Check sheet for the modelled part. Datum: model origin and axes. Units: mm. Face numbers are marked on the shaded views. A direction names the side the tool comes from. Give positions to 0.01 mm unless a question says otherwise; leave off trailing zeros. Order: outer loops, then holes, each group sorted by start corner. A loop starts at its lowest first (then second) coordinate and runs counter-clockwise, first axis right, second up.
```python
from build123d import *

# Parameters (mm, degrees)
SKETCH1_R           = 1.35
BOSS_EXTRUDE1_DEPTH = 3
SKETCH1_3_W         = 89.4
SKETCH1_3_H         = 3
BOSS_EXTRUDE2_DEPTH = 24
CUT_EXTRUDE1_REACH  = 5
SKETCH3_R           = 1.5
SKETCH3_R_2         = 1.75
CUT_EXTRUDE2_START  = -3
SKETCH3_5_R         = 2.25
SKETCH3_5_R_2       = 1.5
CUT_EXTRUDE2_DEPTH  = 1


with BuildPart() as part:
    # Sketch1 → Boss-Extrude1 (new body)
    with BuildSketch(Plane.XY):
        Polygon((-32.2510699, 8.892599614), (-38.2510699, 2.892599614), (-38.2510699, 0.892599614), (51.1489301, 0.892599614), (51.1489301, 2.892599614), (45.1489301, 8.892599614), align=None)
        with Locations((-18.2510699, 4.092599614)):
            Circle(SKETCH1_R, mode=Mode.SUBTRACT)
        with Locations((31.1489301, 4.092599614)):
            Circle(SKETCH1_R, mode=Mode.SUBTRACT)
    extrude(amount=BOSS_EXTRUDE1_DEPTH)

    # Sketch1<3> → Boss-Extrude2 (add)
    with BuildSketch(Plane.XY):
        with Locations((6.4489301, -0.607400386)):
            Rectangle(SKETCH1_3_W, SKETCH1_3_H)
    extrude(amount=BOSS_EXTRUDE2_DEPTH)

    # Sketch3 → Cut-Extrude1 (cut, up to next)
    with BuildSketch(Plane(origin=(0, 0.892599614, 0), x_dir=(1, 0, 0), z_dir=(0, 1, 0)), mode=Mode.PRIVATE) as cut_extrude1_sk1:
        with Locations((48.6489301, -15)):
            Circle(SKETCH3_R)
    cut_extrude1_tool1 = extrude(cut_extrude1_sk1.sketch, amount=-CUT_EXTRUDE1_REACH, mode=Mode.PRIVATE) & part.part
    add(cut_extrude1_tool1.solids().sort_by_distance((48.64893, 0.8926, 15))[0], mode=Mode.SUBTRACT)
    # Sketch3 → Cut-Extrude1 (cut, up to next)
    with BuildSketch(Plane(origin=(0, 0.892599614, 0), x_dir=(1, 0, 0), z_dir=(0, 1, 0)), mode=Mode.PRIVATE) as cut_extrude1_sk2:
        with Locations((48.6489301, -21)):
            Circle(SKETCH3_R)
    cut_extrude1_tool2 = extrude(cut_extrude1_sk2.sketch, amount=-CUT_EXTRUDE1_REACH, mode=Mode.PRIVATE) & part.part
    add(cut_extrude1_tool2.solids().sort_by_distance((48.64893, 0.8926, 21))[0], mode=Mode.SUBTRACT)
    # Sketch3 → Cut-Extrude1 (cut, up to next)
    with BuildSketch(Plane(origin=(0, 0.892599614, 0), x_dir=(1, 0, 0), z_dir=(0, 1, 0)), mode=Mode.PRIVATE) as cut_extrude1_sk3:
        with Locations((-35.7510699, -15)):
            Circle(SKETCH3_R)
    cut_extrude1_tool3 = extrude(cut_extrude1_sk3.sketch, amount=-CUT_EXTRUDE1_REACH, mode=Mode.PRIVATE) & part.part
    add(cut_extrude1_tool3.solids().sort_by_distance((-35.75107, 0.8926, 15))[0], mode=Mode.SUBTRACT)
    # Sketch3 → Cut-Extrude1 (cut, up to next)
    with BuildSketch(Plane(origin=(0, 0.892599614, 0), x_dir=(1, 0, 0), z_dir=(0, 1, 0)), mode=Mode.PRIVATE) as cut_extrude1_sk4:
        with Locations((-35.7510699, -21)):
            Circle(SKETCH3_R)
    cut_extrude1_tool4 = extrude(cut_extrude1_sk4.sketch, amount=-CUT_EXTRUDE1_REACH, mode=Mode.PRIVATE) & part.part
    add(cut_extrude1_tool4.solids().sort_by_distance((-35.75107, 0.8926, 21))[0], mode=Mode.SUBTRACT)
    # Sketch3 → Cut-Extrude1 (cut, up to next)
    with BuildSketch(Plane(origin=(0, 0.892599614, 0), x_dir=(1, 0, 0), z_dir=(0, 1, 0)), mode=Mode.PRIVATE) as cut_extrude1_sk5:
        with Locations((44.5489301, -6.2)):
            Circle(SKETCH3_R_2)
    cut_extrude1_tool5 = extrude(cut_extrude1_sk5.sketch, amount=-CUT_EXTRUDE1_REACH, mode=Mode.PRIVATE) & part.part
    add(cut_extrude1_tool5.solids().sort_by_distance((44.54893, 0.8926, 6.2))[0], mode=Mode.SUBTRACT)
    # Sketch3 → Cut-Extrude1 (cut, up to next)
    with BuildSketch(Plane(origin=(0, 0.892599614, 0), x_dir=(1, 0, 0), z_dir=(0, 1, 0)), mode=Mode.PRIVATE) as cut_extrude1_sk6:
        with Locations((-31.6510699, -6.2)):
            Circle(SKETCH3_R_2)
    cut_extrude1_tool6 = extrude(cut_extrude1_sk6.sketch, amount=-CUT_EXTRUDE1_REACH, mode=Mode.PRIVATE) & part.part
    add(cut_extrude1_tool6.solids().sort_by_distance((-31.65107, 0.8926, 6.2))[0], mode=Mode.SUBTRACT)

    # Sketch3<5> → Cut-Extrude2 (cut)
    with BuildSketch(Plane(origin=(0, 0.892599614, 0), x_dir=(1, 0, 0), z_dir=(0, 1, 0)).offset(CUT_EXTRUDE2_START)):
        with Locations((-35.7510699, -15)):
            Circle(SKETCH3_5_R)
        with Locations((-35.7510699, -15)):
            Circle(SKETCH3_5_R_2, mode=Mode.SUBTRACT)
        with Locations((-35.7510699, -21)):
            Circle(SKETCH3_5_R)
        with Locations((-35.7510699, -21)):
            Circle(SKETCH3_5_R_2, mode=Mode.SUBTRACT)
        with Locations((48.6489301, -15)):
            Circle(SKETCH3_5_R)
        with Locations((48.6489301, -21)):
            Circle(SKETCH3_5_R)
    extrude(amount=CUT_EXTRUDE2_DEPTH, mode=Mode.SUBTRACT)


solid = part.part
```
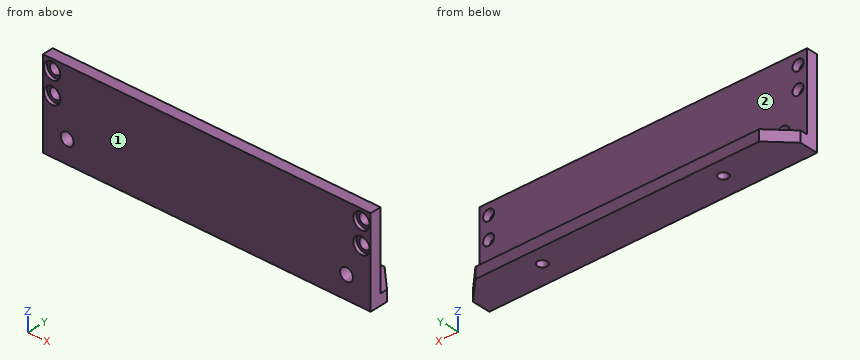
(1) Cross-section at B-B on x = -14.5. Enter the section's corners in (y, z), then the cut area to 3 significant figures.
Response values:
outline: (-2.11, 0) - (8.89, 0) - (8.89, 3) - (0.89, 3) - (0.89, 24) - (-2.11, 24) - close
area: 96.0 mm2
(2) Cross-section at C-C on y = 8. Enter the section's corners in (x, z).
Response values:
outline: (-33.14, 0) - (46.04, 0) - (46.04, 3) - (-33.14, 3) - close
(3) Material ranges on L1, parallel to X at y = -1.7, z = 21; L2, parallel to X at y = -0.25, z = 6.2; L3, parallel to Y at x = -22.5, z = 11.5, recorded low to high.
Response values:
L1: x = -38.25 to -38, -33.5 to 46.4, 50.9 to 51.15
L2: x = -38.25 to -33.4, -29.9 to 42.8, 46.3 to 51.15
L3: y = -2.11 to 0.89
(4) Set-up check for the marked faces 1 and 2: record each of +Z, -Z, +X, -X, +Y, -Y from which the full face is reachable in a straight line by a thin tool's end or side.
Response values:
face 1: +Z, -Z, +X, -X, -Y
face 2: +Z, +X, -X, +Y
(5) Cross-section at A-A on z = 15. Enter the section's corners in (x, y), then the cut area to 3 significant figures.
Response values:
outline: (-38.25, -2.11) - (-38, -2.11) - (-38, -1.11) - (-37.25, -1.11) - (-37.25, 0.89) - (-38.25, 0.89) - close; (-34.25, -1.11) - (-33.5, -1.11) - (-33.5, -2.11) - (46.4, -2.11) - (46.4, -1.11) - (47.15, -1.11) - (47.15, 0.89) - (-34.25, 0.89) - close; (50.15, -1.11) - (50.9, -1.11) - (50.9, -2.11) - (51.15, -2.11) - (51.15, 0.89) - (50.15, 0.89) - close
area: 247 mm2
(6) Gauge pin test, flat ends, axial feed: pin 1 Ø4 at (x, z) = (-35.75, 21) entering from -Y; pin 2 Ø10.5 at (x, z) = (23, 11.5) entering from +Y; pin 3 Ø6 at (x, y) = (37.5, 7.5) entering from +Z. Record the tip position at first contact, or that the pin passes through.
Response values:
pin 1: stops at y = -1.11
pin 2: stops at y = 0.89
pin 3: stops at z = 3
